The listing builds one solid part. Answer for the finished solid, in the listing's coordinates (mm). A direction names the side the tool comes from. Round coordinates to 2 decimals unless told otherwise and drop trailing zeros. Write each loop counter-clockwise with the first axis right and the second up, starting at its lowest first coordinate (ties: lowest second). Pieces come first, ordered by that corner, then holes.
Item 1: Find section A-A on y = 37.5. Give the vertices of the cut face in (x, z), then the cut area to 3 significant figures.
Item 2: Find section B-B on x = 46. Give the vertices of the cut face in (y, z).
Item 3: A tool of negligible diameter and unlimited length cuts with its end or side. For faces 1 (the face through (-10.01, 59.16, 5.92)), 2 (the face through (17.84, 54.76, 4.44)), 3 (the face through (-6.45, 56.82, 26.79)), from which of +Z, -Z, +X, -X, +Y, -Y can it reach the whole face along a straight path? Write none if from no direction.
Item 4: Each of these flat-tipped pins is pushed along its axis until it touches: pin 1 (1.1 mm diameter, centred on x = 46, y = 56, fed in from -Z); pin 2 (2 mm diameter, centred on x = 46, y = 56, fed in from +Z); pin 3 (12 mm diameter, centred on y = 40, z = 20.5, fed in from +X); pin 4 (0.7 mm diameter, centred on x = 17.5, y = 55.5, fed in from -Z). Where does it stop, or does it pass through?
Item 5: Find the intervals of material crossed by probe 1 along X at (y, z) = (56, 10.3); probe 2 along X at (y, z) = (56, 7); probe 3 along Z at (x, y) = (-3.5, 52), in increasing order.
Item 6: For a pull along Y with two mould halves and no side action, classify faces 4 (the face through (42, 30, 11)), 5 (the face through (-10.16, 54.76, 4.44)), 6 (the face through (22, 55, 12)), 7 (the face through (25, 60, 6)) as +Y half, -Y half, draft (parallel to the pull), parting line (faces both ways), or undercut.
```python
from build123d import *

# Parameters (mm, degrees)
PAD_DEPTH       = 12
PAD001_DEPTH    = 30
SKETCH002_R     = 12.9
POCKET_DEPTH    = 35.6974328919
SKETCH003_W     = 100
SKETCH003_H     = 7
POCKET001_DEPTH = 23
SKETCH004_R     = 0.9
POCKET002_DEPTH = 12
SKETCH005_R     = 1.25
POCKET003_DEPTH = 9
POCKET004_DEPTH = 23


with BuildPart() as part:
    # Sketch → Pad (new body)
    with BuildSketch(Plane.XY):
        with BuildLine():
            Line((33.5410196625, 30), (50, 30))
            Line((50, 30), (50, 60))
            Line((0, 60), (50, 60))
            ThreePointArc((0, 60), (-10.1461187235, 59.1359135792), (-20, 56.5685424949))
            Line((-20, 40.3112887415), (-20, 56.5685424949))
            ThreePointArc((33.5410196625, 30), (8.5100218715, 44.1880020792), (-20, 40.3112887415))
        make_face()
    extrude(amount=PAD_DEPTH)

    # Sketch001 → Pad001 (new body)
    with BuildSketch(Plane.XY.offset(12)):
        Polygon((-4.671183324, 62.6409760428), (29.7557878907, 52.1155946728), (26.247327434, 40.6399376012), (-8.1796437806, 51.1653189712), align=None)
    extrude(amount=PAD001_DEPTH)

    # Sketch002 → Pocket (cut, through all)
    with BuildSketch(Plane(origin=(17.1148962148, 55.9803030991, 0), x_dir=(-0.956304756, 0.2923717047, 0), z_dir=(0.2923717047, 0.956304756, 0))):
        with Locations((4.7815237798, 42)):
            Circle(SKETCH002_R)
    extrude(amount=-POCKET_DEPTH, mode=Mode.SUBTRACT)

    # Sketch003 → Pocket001 (cut)
    with BuildSketch(Plane.XZ.offset(-30)):
        with Locations((11.7941241648, 5.5)):
            Rectangle(SKETCH003_W, SKETCH003_H)
    extrude(amount=-POCKET001_DEPTH, mode=Mode.SUBTRACT)

    # Sketch004 → Pocket002 (cut)
    with BuildSketch(Plane(origin=(0, 0, 0), x_dir=(1, 0, 0), z_dir=(0, 0, -1))):
        with Locations((-10, -56)):
            Circle(SKETCH004_R)
        with Locations((18, -56)):
            Circle(SKETCH004_R)
        with Locations((46, -56)):
            Circle(SKETCH004_R)
    extrude(amount=-POCKET002_DEPTH, mode=Mode.SUBTRACT)

    # Sketch005 → Pocket003 (cut)
    with BuildSketch(Plane(origin=(0, 0, 0), x_dir=(1, 0, 0), z_dir=(0, 0, -1))):
        with Locations((18, -56)):
            Circle(SKETCH005_R)
        with Locations((-10, -56)):
            Circle(SKETCH005_R)
        with Locations((46, -56)):
            Circle(SKETCH005_R)
    extrude(amount=-POCKET003_DEPTH, mode=Mode.SUBTRACT)

    # Sketch006 → Pocket004 (cut)
    with BuildSketch(Plane.XZ.offset(-30)):
        Polygon((71.676384, 11.631999), (1.884626, 7.843544), (1.884626, 3.12902), (71.676384, 0.519198), align=None)
    extrude(amount=-POCKET004_DEPTH, mode=Mode.SUBTRACT)


solid = part.part
```
Check values:
1. outline: (24.87, 0) - (50, 0) - (50, 1.33) - (32.08, 2) - (24.87, 2) - close; (24.87, 9.09) - (50, 10.46) - (50, 12) - (24.87, 12) - close
1. area: 100 mm2
2. outline: (30, 0) - (54.75, 0) - (54.75, 9) - (55.1, 9) - (55.1, 12) - (30, 12) - (30, 10.24) - (53, 10.24) - (53, 1.48) - (30, 1.48) - close; (56.9, 9) - (57.25, 9) - (57.25, 0) - (60, 0) - (60, 12) - (56.9, 12) - close
3. face 1: -Z, -X, +Y
3. face 2: -Z
3. face 3: +Z, -X, +Y
4. pin 1: passes through
4. pin 2: stops at z = 12
4. pin 3: stops at x = 27.89
4. pin 4: stops at z = 9
5. probe 1: x = -20 to -10.9, -9.1 to 17.1, 18.9 to 45.1, 46.9 to 50
5. probe 2: x = -20 to -11.25, -8.75 to 16.75, 19.25 to 44.75, 47.25 to 50
5. probe 3: z = 0 to 2, 9 to 42
6. face 4: -Y half
6. face 5: undercut
6. face 6: draft
6. face 7: +Y half
